from build123d import *

# Parameters (mm, degrees)
BOSS_EXTRUDE1_DEPTH = 3.8
SKETCH2_W           = 11
SKETCH2_H           = 2.8
BOSS_EXTRUDE2_DEPTH = 7
SKETCH3_W           = 4
SKETCH3_H           = 8.4
CUT_EXTRUDE1_DEPTH  = 43.932622105
SKETCH4_W           = 11
SKETCH4_H           = 2.4
BOSS_EXTRUDE3_DEPTH = 2.2
SKETCH5_W           = 5
SKETCH5_H           = 2.4
BOSS_EXTRUDE4_DEPTH = 4
SKETCH6_W           = 9
SKETCH6_H           = 2.8
BOSS_EXTRUDE5_DEPTH = 2.8
SKETCH7_W           = 2.8
SKETCH7_H           = 6.6
BOSS_EXTRUDE6_DEPTH = 4
SKETCH8_W           = 4.732050808
SKETCH8_H           = 1
CUT_EXTRUDE2_DEPTH  = 44.13200715
SKETCH9_W           = 4.732050807
SKETCH9_H           = 1
CUT_EXTRUDE3_DEPTH  = 44.13200715
SKETCH10_W          = 2
SKETCH10_H          = 3
CUT_EXTRUDE4_DEPTH  = 43.932622105
DRAFT1_ANGLE        = 60
CHAMFER1_SIZE       = 0.6
FILLET1_R           = 1.2


with BuildPart() as part:
    # Sketch1 → Boss-Extrude1 (new body)
    with BuildSketch(Plane(origin=(0, 6.6, 0), x_dir=(1, 0, 0), z_dir=(0, 1, 0))):
        Polygon((-21.625238963, 0.4), (-24.025238963, 2.8), (-40.625238963, 2.8), (-40.625238963, 0), (-21.625238963, 0), align=None)
    extrude(amount=-BOSS_EXTRUDE1_DEPTH)

    # Sketch2 → Boss-Extrude2 (add)
    with BuildSketch(Plane(origin=(0, 6.6, 0), x_dir=(-1, 0, 0), z_dir=(0, 1, 0))):
        with Locations((35.125238963, -1.4)):
            Rectangle(SKETCH2_W, SKETCH2_H)
    extrude(amount=BOSS_EXTRUDE2_DEPTH)

    # Sketch3 → Cut-Extrude1 (cut, through all)
    with BuildSketch(Plane.XY):
        with Locations((-38.625238963, 7)):
            Rectangle(SKETCH3_W, SKETCH3_H)
    extrude(amount=-CUT_EXTRUDE1_DEPTH, mode=Mode.SUBTRACT)

    # Sketch4 → Boss-Extrude3 (add)
    with BuildSketch(Plane(origin=(0, 0, -2.8), x_dir=(-1, 0, 0), z_dir=(0, 0, -1))):
        with Locations((35.125238963, 12.4)):
            Rectangle(SKETCH4_W, SKETCH4_H)
    extrude(amount=BOSS_EXTRUDE3_DEPTH)

    # Sketch5 → Boss-Extrude4 (add)
    with BuildSketch(Plane(origin=(-29.625238963, 0, 0), x_dir=(0, 0, -1), z_dir=(1, 0, 0))):
        with Locations((2.5, 12.4)):
            Rectangle(SKETCH5_W, SKETCH5_H)
    extrude(amount=BOSS_EXTRUDE4_DEPTH)

    # Sketch6 → Boss-Extrude5 (add)
    with BuildSketch(Plane.XZ.offset(-2.8)):
        with Locations((-32.125238963, -1.4)):
            Rectangle(SKETCH6_W, SKETCH6_H)
    extrude(amount=BOSS_EXTRUDE5_DEPTH)

    # Sketch7 → Boss-Extrude6 (add)
    with BuildSketch(Plane.ZY.offset(36.625238963)):
        with Locations((-1.4, 3.3)):
            Rectangle(SKETCH7_W, SKETCH7_H)
    extrude(amount=BOSS_EXTRUDE6_DEPTH)

    # Sketch8 → Cut-Extrude2 (cut, through all)
    with BuildSketch(Plane(origin=(0, 0, -5), x_dir=(-1, 0, 0), z_dir=(0, 0, -1))):
        with Locations((38.259213559, 13.1)):
            Rectangle(SKETCH8_W, SKETCH8_H)
    extrude(amount=-CUT_EXTRUDE2_DEPTH, mode=Mode.SUBTRACT)

    # Sketch9 → Cut-Extrude3 (cut, through all)
    with BuildSketch(Plane.XY):
        with Locations((-27.991264367, 13.1)):
            Rectangle(SKETCH9_W, SKETCH9_H)
    extrude(amount=-CUT_EXTRUDE3_DEPTH, mode=Mode.SUBTRACT)

    # Sketch10 → Cut-Extrude4 (cut, through all)
    with BuildSketch(Plane(origin=(0, 0, -2.8), x_dir=(-1, 0, 0), z_dir=(0, 0, -1))):
        with Locations((39.625238963, 4.3)):
            Rectangle(SKETCH10_W, SKETCH10_H)
    extrude(amount=-CUT_EXTRUDE4_DEPTH, mode=Mode.SUBTRACT)

    # Draft1
    draft1_faces = [part.faces().sort_by_distance(p)[0] for p in [
        (-30.35728977, 13.1, -2.5),
        (-35.893188155, 13.1, -2.5),
    ]]
    draft(draft1_faces, Plane.ZX.offset(13.6), DRAFT1_ANGLE)

    # Chamfer1
    chamfer1_edges = [part.edges().sort_by_distance(p)[0] for p in [
        (-33.125238963, 11.2, -5),
    ]]
    chamfer(chamfer1_edges, length=CHAMFER1_SIZE)

    # Fillet1
    fillet1_edges = [part.edges().sort_by_distance(p)[0] for p in [
        (-25.625238963, 12.2, -5),
        (-25.625238963, 11.9, 0),
        (-40.625238963, 12.2, -5),
        (-40.625238963, 11.9, 0),
    ]]
    fillet(fillet1_edges, radius=FILLET1_R)


solid = part.part
The model under review builds one solid part; all positions refer to its coordinate system, in mm. A direction names the side the tool comes from. Round coordinates to 2 decimals unless told otherwise and drop trailing zeros. Write each loop counter-clockwise with the first axis right and the second up, starting at its lowest first coordinate (ties: lowest second). Pieces come first, ordered by that corner, then holes. Notation, with made-up numbers: M 57.25,-23 L 77.25,-23 A18 cw 77.25,-6 Z; hole C 23.25,50.5 d6. An arc over 180 degrees is marked long. Use a Markdown table: item, result. Add a question column.
Q1. We need section B-B, the plane z = -3.25. State the section outline as (x, y) points, plus the area to 3 significant figures.
Q2. We need section D-D, the plane y = 6. State the section outline as (x, z) points, plus the area to 3 significant figures.
Q3. To check wall thickness, follow line 1 (Y direction, x = -39.25, z = -0.85); line 2 (Z direction, x = -35.75, y = 10.75); line 3 (X direction, y = 8.5, z = -2.6). State the ranges of each line that lie inside material, in increasing order.
Q4. The part is to be moulded in two halves that separate along Y. For faces 6 (the face through (-39, 6.6, -1)), 7 (the face through (-22.808, 4.727, -1.583)), 8 (the face through (-27, 12.6, -2)), say which applies: pulls with the +Y half, pulls with the -Y half, needs draft (parallel to the pull), parting line crosses it, or undercut.
Q5. Insertion check: pin 1 (0.8 mm diameter, centred on y = 4.5, z = -1.5, fed in from -X); pin 2 (3 mm diameter, centred on y = 2, z = -1.5, fed in from +X); pin 3 (1.4 mm diameter, centred on x = -24.5, z = -1, fed in from +Y); pin 4 (2 mm diameter, centred on y = 8, z = -1, fed in from -X). Each pin has a flat end and moves straight along its axis. Give the tip position at first contact, or say it passes through.
Q6. We need section C-C, the plane x = -26.5. State the section outline as (y, z) points, plus the area to 3 significant figures.
Q7. Machinability: for faces 1 (the face through (-29.625, 9, -1)), 2 (the face through (-40.26, 11.89, -0.34)), 3 (the face through (-36.625, 9, -1)), 4 (the face through (-25, 2.8, -1)), 5 (the face through (-33, 11.2, -3)), which of the approach directions +Z, -Z, +X, -X, +Y, -Y give a long, thin tool a straight path to every point of the face, cutting with its end or side? Answer none if there is none.
Q8. We need section A-A, the plane x = -34.25. State the section outline as (y, z) points.
Findings below:
| question | item | result |
|---|---|---|
| 1 | outline | M -40.63,11.2 L -25.63,11.2 L -25.63,12.6 L -28.63,12.6 L -30.36,13.6 L -35.89,13.6 L -37.63,12.6 L -40.63,12.6 Z |
| 1 | area | 28.3 mm² |
| 2 | outline | M -40.63,-2.8 L -24.03,-2.8 L -21.63,-0.4 L -21.63,0 L -40.63,0 Z |
| 2 | area | 50.3 mm² |
| 3 | line 1 | y = 0 to 2.8, 5.8 to 6.6, 11.2 to 12.6 |
| 3 | line 2 | z = -2.8 to 0 |
| 3 | line 3 | x = -36.63 to -29.63 |
| 4 | face 6 | undercut |
| 4 | face 7 | needs draft |
| 4 | face 8 | pulls with the +Y half |
| 5 | pin 1 | stops at x = -38.63 |
| 5 | pin 2 | stops at x = -21.63 |
| 5 | pin 3 | stops at y = 6.6 |
| 5 | pin 4 | stops at x = -36.63 |
| 6 | outline | M 2.8,-2.8 L 6.6,-2.8 L 6.6,0 L 2.8,0 Z; M 11.2,-4.4 L 11.76,-4.96 L 12.6,-4.96 L 12.6,-0.04 L 11.2,-0.04 Z |
| 6 | area | 17.4 mm² |
| 7 | face 1 | +Z, -Z, +X |
| 7 | face 2 | +Z, -X, +Y |
| 7 | face 3 | +Z, -Z, -X |
| 7 | face 4 | +Z, -Z, +X, -Y |
| 7 | face 5 | -Z |
| 8 | outline | M 0,-2.8 L 11.2,-2.8 L 11.2,-4.4 L 11.8,-5 L 13.6,-5 L 13.6,0 L 0,0 Z |
